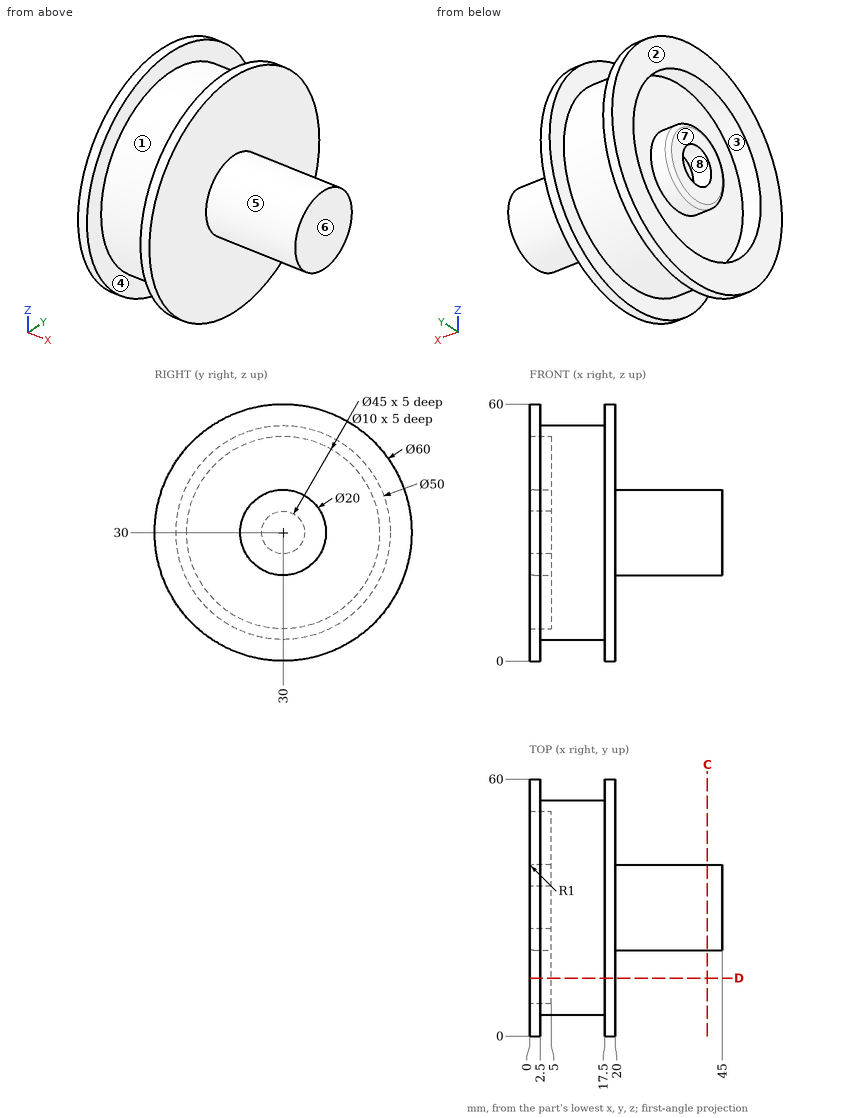
Drawing for the job (mm, zero at the part's lowest x, y, z). A direction names the side the tool comes from. Give positions to 0.01 mm unless a question says otherwise; leave off trailing zeros. Order: outer loops, then holes, each group sorted by start corner. A loop starts at its lowest first (then second) coordinate and runs counter-clockwise, first axis right, second up. Notation, with made-up numbers: M -4,52.5 L 40,52.5 A17 ccw 40,77.5 Z; hole C 77.25,80.5 d4. An arc over 180 degrees is marked long. Use a Markdown table: item, result. Add a question column.
(1) Saw through at C-C, the plane x = 41.5. Give the cut face in (y, z), and give its area (3 significant figures).
(2) 3-axis set-ups, long thin cutter, end or side, ignore diameter. For the marked faces 4, 5, 6, 7 and 8: which of +Z, -Z, +X, -X, +Y, -Y reach the whole face in a straight line?
(3) Drop flat-ended pins along their axis: P1, Ø8, axis at y = 16, z = 47, coming from the +X side; P2, Ø6, axis at x = 20, y = 26, coming from the +Z side; P3, Ø12, axis at x = 37.5, z = 22.5, coming from the -Y side. Give the stop position or say it passes through.
(4) Probe line 1 along Z through (x, y) = (1.85, 30); line 2 along Z through (x, y) = (3.6, 30); line 3 along X through (y, z) = (38, 3). List the from-to ranges inside material, lowest first. Write a range as [from, to].
(5) Mould opens along Y. For the marked faces 1, 2 and 3 say: +Y half, -Y half, draft (parallel to the pull), parting line (faces both ways), or undercut.
(6) Saw through at D-D, the plane y = 13.5. Give the cut face in (x, z), and give its area (3 significant figures).
Answer key:
| question | item | result |
|---|---|---|
| 1 | outline | C 30,30 d20 |
| 1 | area | 314 mm^2 |
| 2 | face 4 | none |
| 2 | face 5 | +X |
| 2 | face 6 | +Z, -Z, +X, +Y, -Y |
| 2 | face 7 | +Z, -Z, -X, +Y, -Y |
| 2 | face 8 | -X |
| 3 | P1 | x = 20 |
| 3 | P2 | z = 59.98 |
| 3 | P3 | y = 20.11 |
| 4 | line 1 | [0, 7.5], [20, 25], [35, 40], [52.5, 60] |
| 4 | line 2 | [5, 7.5], [20, 25], [35, 40], [52.5, 55] |
| 4 | line 3 | [0, 2.5], [17.5, 20] |
| 5 | face 1 | parting line |
| 5 | face 2 | draft |
| 5 | face 3 | undercut |
| 6 | outline | M 0,4.95 L 2.5,4.95 L 2.5,11.22 L 17.5,11.22 L 17.5,4.95 L 20,4.95 L 20,55.05 L 17.5,55.05 L 17.5,48.78 L 2.5,48.78 L 2.5,55.05 L 0,55.05 L 0,45.3 L 5,45.3 L 5,14.7 L 0,14.7 Z |
| 6 | area | 661 mm^2 |
